from build123d import *

# Parameters (mm, degrees)
ESKIZ_KONTUR_W        = 3.2
ESKIZ_KONTUR_H        = 8.2
PLASTINA_DEPTH        = 3
OTVERSTIYA_DEPTH      = 49.541218109
OTVERSTIYA_DEPTH_BACK = 49.541218109
ESKIZ_OTVERSTIYA_R    = 4.5
ESKIZ_OTVERSTIYA_R_2  = 1.65


with BuildPart() as part:
    # Eskiz_kontur → Plastina (new body)
    with BuildSketch(Plane.XY):
        with BuildLine():
            Line((41.499998426, -24.999999723), (25.999998426, -24.999999723))
            Line((25.999998426, -24.999999723), (-4.976321574, -10.919529723))
            ThreePointArc((-4.976321574, -10.919529723), (-11.817691954, 2.083782335), (-0.94151, 11.96301))
            Line((-0.94151, 11.96301), (26, 14))
            Line((26, 14), (41.499998426, 14))
            Line((41.499998426, 14), (41.499998426, -24.999999723))
        make_face()
        with Locations((36.5, -16)):
            Rectangle(ESKIZ_KONTUR_W, ESKIZ_KONTUR_H, mode=Mode.SUBTRACT)
        with Locations((36.5, 6)):
            Rectangle(ESKIZ_KONTUR_W, ESKIZ_KONTUR_H, mode=Mode.SUBTRACT)
    extrude(amount=PLASTINA_DEPTH)

    # Eskiz_otverstiya → Otverstiya (cut, two sides: drawn at the far end of the back side and taken through both)
    with BuildSketch(Plane.XY.offset(-OTVERSTIYA_DEPTH_BACK)):
        with Locations((17, -8)):
            Circle(ESKIZ_OTVERSTIYA_R)
        Circle(ESKIZ_OTVERSTIYA_R_2)
        with Locations((36.5, -5)):
            Circle(ESKIZ_OTVERSTIYA_R_2)
    extrude(amount=OTVERSTIYA_DEPTH + OTVERSTIYA_DEPTH_BACK, mode=Mode.SUBTRACT)


solid = part.part
Can you work these out from the model? Positions are in its coordinate system, mm. A direction names the side the tool comes from. Give positions to 0.01 mm unless a question says otherwise; leave off trailing zeros. Loops run counter-clockwise (first coordinate to the right, second up) from the corner with the lowest first, then second, coordinate; pieces in that order, holes last. Notation, with made-up numbers: M 18.25,40 L 38.25,40 A16 ccw 38.25,66 Z; hole C 31,-1.5 d5. An arc over 180 degrees is marked long. One line per item, written item: value.
1) I'm going to push flat-ended pins straight in: pin 1 (1.5 mm diameter, centred on y = 5, z = 1.5, fed in from -X); pin 2 (3 mm diameter, centred on x = 36.5, y = -5, fed in from -Z); pin 3 (1.5 mm diameter, centred on x = 11, z = 0.5, fed in from -Y); pin 4 (1.5 mm diameter, centred on y = -16, z = 2, fed in from -X). Where does each tip first touch, or does it pass through?
Geometry check:
pin 1: stops at x = -11.22
pin 2: passes through
pin 3: stops at y = -18.52
pin 4: stops at x = 4.55
2) Imagine slicing it at D-D on x = 17. Write out the boundary of the cut face in (y, z).
Geometry check:
outline: M -20.91,0 L -12.5,0 L -12.5,3 L -20.91,3 Z; M -3.5,0 L 13.32,0 L 13.32,3 L -3.5,3 Z
3) Thinking about a two-plate mould opening in Y: for faces 3 (the face through (12.341, 12.967, 1.479)), 4 (the face through (36, 1.9, 1)), 5 (the face through (34.9, 6, 1)), 6 (the face through (34, -25, 1)), which applies, +Y half, -Y half, draft (parallel to the pull), parting line (faces both ways), or undercut?
Geometry check:
face 3: +Y half
face 4: undercut
face 5: undercut
face 6: -Y half
4) Imagine slicing it at B-B on x = 36.5. Write out the boundary of the cut face in (y, z), and give its area (3 significant figures).
Geometry check:
outline: M -25,0 L -20.1,0 L -20.1,3 L -25,3 Z; M -11.9,0 L -6.65,0 L -6.65,3 L -11.9,3 Z; M -3.35,0 L 1.9,0 L 1.9,3 L -3.35,3 Z; M 10.1,0 L 14,0 L 14,3 L 10.1,3 Z
area: 57.9 mm²
5) Imagine slicing it at C-C on z = 2.2. Write out the boundary of the cut face in (x, y), and give its area (3 significant figures).
Geometry check:
outline: M -4.98,-10.92 L 26,-25 L 41.5,-25 L 41.5,14 L 26,14 L -0.94,11.96 A12 ccw Z; hole C 0,0 d3.3; hole C 17,-8 d9; hole C 36.5,-5 d3.3; hole M 34.9,-20.1 L 38.1,-20.1 L 38.1,-11.9 L 34.9,-11.9 Z; hole M 34.9,1.9 L 38.1,1.9 L 38.1,10.1 L 34.9,10.1 Z
area: 1,530 mm²
6) Imagine slicing it at A-A on y = 0. Write out the boundary of the cut face in (x, z).
Geometry check:
outline: M -12,0 L -1.65,0 L -1.65,3 L -12,3 Z; M 1.65,0 L 41.5,0 L 41.5,3 L 1.65,3 Z
7) Please list where these lines run through material, in increasing order: line 1 (Y direction, x = 36.5, z = 1.3); line 2 (X direction, y = -5, z = 2.2); line 3 (X direction, y = -4, z = 1).
Geometry check:
line 1: y = -25 to -20.1, -11.9 to -6.65, -3.35 to 1.9, 10.1 to 14
line 2: x = -10.91 to 13.65, 20.35 to 34.85, 38.15 to 41.5
line 3: x = -11.31 to 14.94, 19.06 to 35.19, 37.81 to 41.5
8) On a 3-axis mill with a long thin cutter (end or side, diameter ignored), from which of +Z, -Z, +X, -X, +Y, -Y can I reach the whole of each face in a straight line? I mean faces 1 (the face through (38.1, 6, 1)), 2 (the face through (21, -5, 3)). Say none if no direction works.
Geometry check:
face 1: +Z, -Z
face 2: +Z, +X, -X, +Y, -Y
